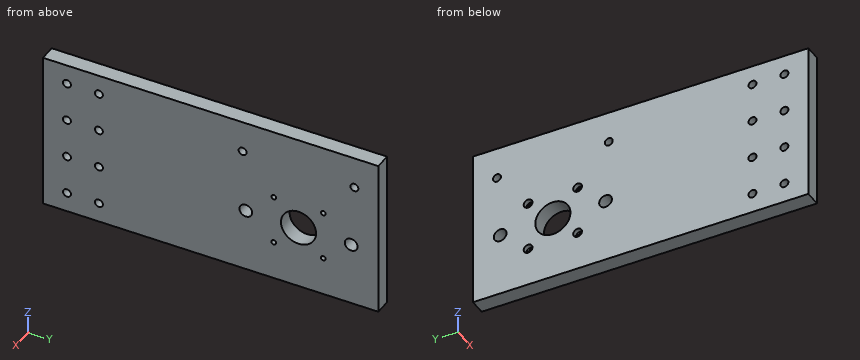
```python
from build123d import *

# Parameters (mm, degrees)
SKETCH2_W                       = 100
SKETCH2_H                       = 210
SKETCH2_R                       = 4
BOSS_EXTRUDE1_DEPTH             = 10
SKETCH3_R                       = 2.5
MOUNT_DEPTH                     = 11
SKETCH7_R                       = 2.5
SUPPORT_PROFILE_MOUNT_DEPTH     = 11
SKETCH4_R                       = 11
SKETCH4_R_2                     = 1.5
STEPPER_MOUNT_DEPTH             = 11
SKETCH6_R                       = 2.75
STEPPER_MOUNT_COUNTERSINK_DEPTH = 3


with BuildPart() as part:
    # Sketch2 → Boss-Extrude1 (new body)
    with BuildSketch(Plane(origin=(0, 0, 0), x_dir=(0, 0, -1), z_dir=(1, 0, 0))):
        with Locations((-10, 0)):
            Rectangle(SKETCH2_W, SKETCH2_H)
        with Locations((0, 88)):
            Circle(SKETCH2_R, mode=Mode.SUBTRACT)
        with Locations((0, 22)):
            Circle(SKETCH2_R, mode=Mode.SUBTRACT)
    extrude(amount=BOSS_EXTRUDE1_DEPTH)

    # Sketch3 → mount (cut, through all)
    with BuildSketch(Plane(origin=(10, 0, 0), x_dir=(0, 0, -1), z_dir=(1, 0, 0))):
        with Locations((-22.5, -70)):
            Circle(SKETCH3_R)
        with Locations((-47.5, -70)):
            Circle(SKETCH3_R)
        with Locations((-47.5, -90)):
            Circle(SKETCH3_R)
        with Locations((-22.5, -90)):
            Circle(SKETCH3_R)
        with Locations((2.5, -90)):
            Circle(SKETCH3_R)
        with Locations((27.5, -90)):
            Circle(SKETCH3_R)
        with Locations((27.5, -70)):
            Circle(SKETCH3_R)
        with Locations((2.5, -70)):
            Circle(SKETCH3_R)
    extrude(amount=-MOUNT_DEPTH, mode=Mode.SUBTRACT)

    # Sketch7 → support_profile_mount (cut, through all)
    with BuildSketch(Plane(origin=(10, 0, 0), x_dir=(0, 0, -1), z_dir=(1, 0, 0))):
        with Locations((-40, 90)):
            Circle(SKETCH7_R)
        with Locations((-40, 20)):
            Circle(SKETCH7_R)
    extrude(amount=-SUPPORT_PROFILE_MOUNT_DEPTH, mode=Mode.SUBTRACT)

    # Sketch4 → stepper_mount (cut, through all)
    with BuildSketch(Plane(origin=(10, 0, 0), x_dir=(0, 0, -1), z_dir=(1, 0, 0))):
        with Locations((0, 55)):
            Circle(SKETCH4_R)
        with Locations((-15.5, 70.5)):
            Circle(SKETCH4_R_2)
        with Locations((15.5, 70.5)):
            Circle(SKETCH4_R_2)
        with Locations((-15.5, 39.5)):
            Circle(SKETCH4_R_2)
        with Locations((15.5, 39.5)):
            Circle(SKETCH4_R_2)
    extrude(amount=-STEPPER_MOUNT_DEPTH, mode=Mode.SUBTRACT)

    # Sketch6 → stepper_mount_countersink (cut)
    with BuildSketch(Plane.ZY):
        with Locations((-15.5, 70.5)):
            Circle(SKETCH6_R)
        with Locations((15.5, 70.5)):
            Circle(SKETCH6_R)
        with Locations((15.5, 39.5)):
            Circle(SKETCH6_R)
        with Locations((-15.5, 39.5)):
            Circle(SKETCH6_R)
    extrude(amount=-STEPPER_MOUNT_COUNTERSINK_DEPTH, mode=Mode.SUBTRACT)


solid = part.part
```
Input: part model. Units: mm. Frame: model coordinates. Coordinates: 2 decimals unless noted, no trailing zeros. Write each loop counter-clockwise with the first axis right and the second up, starting at its lowest first coordinate (ties: lowest second). Pieces come first, ordered by that corner, then holes. Notation, with made-up numbers: (42, -31.75) -> (58, -31.75) arc R9 ccw to (58, -25.75) -> close; hole circle Ø6 at (-36, 1). An arc over 180 degrees is marked (long way). Answer as a JSON object with one key per item and string values.
1. Section B-B on z = 47.5. Return the cut outline in (x, y).
Result set:
{"outline": "(0, -105) -> (10, -105) -> (10, -92.5) -> (0, -92.5) -> close; (0, -87.5) -> (10, -87.5) -> (10, -72.5) -> (0, -72.5) -> close; (0, -67.5) -> (10, -67.5) -> (10, 105) -> (0, 105) -> close"}
2. Section A-A on y = -70. Return the cut outline in (x, z).
Result set:
{"outline": "(0, -40) -> (10, -40) -> (10, -30) -> (0, -30) -> close; (0, -25) -> (10, -25) -> (10, -5) -> (0, -5) -> close; (0, 0) -> (10, 0) -> (10, 20) -> (0, 20) -> close; (0, 25) -> (10, 25) -> (10, 45) -> (0, 45) -> close; (0, 50) -> (10, 50) -> (10, 60) -> (0, 60) -> close"}
3. Section C-C on x = 5. Count the separate pieces of the cut face and the enclosed holes in it, then the cut area to 3 significant figures.
Result set:
{"separate pieces": "1", "enclosed holes": "17", "area": "20,300 mm2"}
4. First-contact query: P1, Ø5, axis at y = 39.5, z = 15.5, coming from the -X side. Flat tip, straight axial feed; report the tip coordinate or a pass-through.
Result set:
{"P1": "stops at x = 3"}
5. Section D-D on y = 20. Return the cut outline in (x, z).
Result set:
{"outline": "(0, -40) -> (10, -40) -> (10, -3.46) -> (0, -3.46) -> close; (0, 3.46) -> (10, 3.46) -> (10, 37.5) -> (0, 37.5) -> close; (0, 42.5) -> (10, 42.5) -> (10, 60) -> (0, 60) -> close"}
6. Material intervals for line 1 (Y direction, x = 3, z = 47.5); line 2 (Y direction, x = 7.5, z = -15.5); line 3 (Y direction, x = 3.75, z = -2.5), sorted ascending. Write a range as from..to.
Result set:
{"line 1": "y = -105..-92.5, -87.5..-72.5, -67.5..105", "line 2": "y = -105..38, 41..69, 72..105", "line 3": "y = -105..-92.5, -87.5..-72.5, -67.5..18.88, 25.12..44.29, 65.71..84.88, 91.12..105"}
